Could you check a few things on this drawing? It's one solid part, dimensions in mm from its lowest x, y, z. A direction names the side the tool comes from. Round coordinates to 2 decimals unless told otherwise and drop trailing zeros. Write each loop counter-clockwise with the first axis right and the second up, starting at its lowest first coordinate (ties: lowest second). Pieces come first, ordered by that corner, then holes. Notation, with made-up numbers: (21.5, -16.75) - (59.5, -16.75) arc R9 cw to (59.5, -12.75) - close; hole circle Ø11 at (10, 62.25). An arc over 180 degrees is marked (long way). Put each result on its own line as item: value.
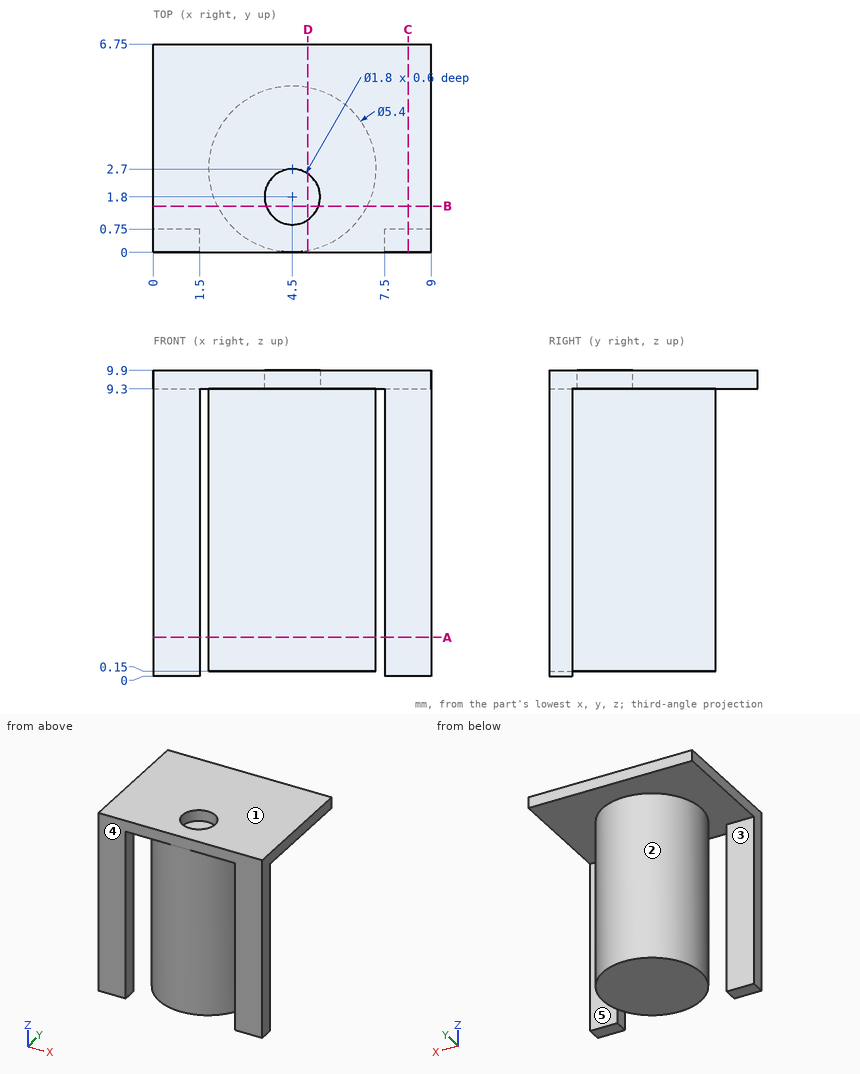
(1) I'm going to push flat-ended pins straight in: pin 1 (3 mm diameter, centred on y = 1, z = 3.5, fed in from +X); pin 2 (2 mm diameter, centred on x = 2.5, z = 6.5, fed in from +Y); pin 3 (1.6 mm diameter, centred on x = 8.5, z = 5.5, fed in from +Y); pin 4 (1.6 mm diameter, centred on x = 4, y = 2, fed in from -Z). Where does each tip first touch, or does it pass through?
Values found:
pin 1: stops at x = 9
pin 2: stops at y = 5.21
pin 3: stops at y = 0.75
pin 4: stops at z = 0.15
(2) Imagine slicing it at A-A, the plane z = 1.25. List the corners of the cut face in (x, y) for me.
Values found:
outline: (0, 0) - (1.5, 0) - (1.5, 0.75) - (0, 0.75) - close; circle Ø5.4 at (4.5, 2.7); (7.5, 0) - (9, 0) - (9, 0.75) - (7.5, 0.75) - close
(3) Imagine slicing it at C-C, the plane x = 8.25. List the corners of the cut face in (y, z) for me, then the cut area to 3 significant figures.
Values found:
outline: (0, 0) - (0.75, 0) - (0.75, 9.3) - (6.75, 9.3) - (6.75, 9.9) - (0, 9.9) - close
area: 11.0 mm^2
(4) Imagine slicing it at D-D, the plane x = 5. List the corners of the cut face in (y, z) for me, then the cut area to 3 significant figures.
Values found:
outline: (0, 9.3) - (0.05, 9.3) - (0.05, 0.15) - (5.35, 0.15) - (5.35, 9.3) - (6.75, 9.3) - (6.75, 9.9) - (2.55, 9.9) - (2.55, 9.3) - (1.05, 9.3) - (1.05, 9.9) - (0, 9.9) - close
area: 51.7 mm^2
(5) For the marked faces 3, 4 and 5, which set-ups out of +Z, -Z, +X, -X, +Y, -Y let a thin tool reach every point of the face, with its end or its side?
Values found:
face 3: -Z, -X, +Y
face 4: +Z, -Z, +X, -X, -Y
face 5: -Z, +X, +Y
(6) Please list where these lines run through material, in increasing order: probe 1 along Y at (x, z) = (4.5, 9.7); probe 2 along Z at (x, y) = (1, 2.75); probe 3 along Z at (x, y) = (4, 0.75). Write a range as from..to.
Values found:
probe 1: y = 0..0.9, 2.7..6.75
probe 2: z = 9.3..9.9
probe 3: z = 0.15..9.9
(7) If we mould it in two halves opening along X, with no side actions, what happens to the marked faces 1 and 2? For each: pulls with the +X half, pulls with the -X half, needs draft (parallel to the pull), parting line crosses it, or undercut.
Values found:
face 1: needs draft
face 2: undercut
(8) Imagine slicing it at B-B, the plane y = 1.5. List the corners of the cut face in (x, z) for me.
Values found:
outline: (0, 9.3) - (2.08, 9.3) - (2.08, 0.15) - (6.92, 0.15) - (6.92, 9.3) - (9, 9.3) - (9, 9.9) - (5.35, 9.9) - (5.35, 9.3) - (3.65, 9.3) - (3.65, 9.9) - (0, 9.9) - close
